Verification items for this drawing (mm, ordinates from the low corner). A direction names the side the tool comes from. Round coordinates to 2 decimals unless told otherwise and drop trailing zeros. Loops run counter-clockwise (first coordinate to the right, second up) from the corner with the lowest first, then second, coordinate; pieces in that order, holes last. Notation, with made-up numbers: (83.25, 12.5) -> (108.25, 12.5) arc R8 cw to (108.25, 21.5) -> close; hole circle Ø3 at (-7.75, 82). An arc over 180 degrees is marked (long way). One line per item, written item: value. Start each with the question number.
1. Cross-section at D-D on z = 41.5. Record the cut outline in (x, y), then the cut area to 3 significant figures.
2. Cross-section at C-C on z = 66. Record the cut outline in (x, y).
3. Material ranges on L1, parallel to Z at x = 33.5, y = 19.5; L2, parallel to X at y = 18, z = 29 (3 decimals); L3, parallel to Y at x = 28, z = 39, recorded low to high.
4. Go/stop test with flat-tipped pins: pin 1 (3 mm diameter, centred on x = 30, z = 19.5, fed in from +Y); pin 2 (5 mm diameter, centred on x = 11.5, y = 20.5, fed in from -Z); pin 3 (6 mm diameter, centred on x = 20.5, z = 18, fed in from +Y); pin 4 (4 mm diameter, centred on y = 25.5, z = 58, fed in from -X). Record where each tip stops, or that it passes through.
5. Set-up check for the marked faces 1, 2 and 3: record each of +Z, -Z, +X, -X, +Y, -Y from which the full face is reachable in a straight line by a thin tool's end or side.
6. Cross-section at A-A on x = 18.75. Record the cut outline in (y, z), then the cut area to 3 significant figures.
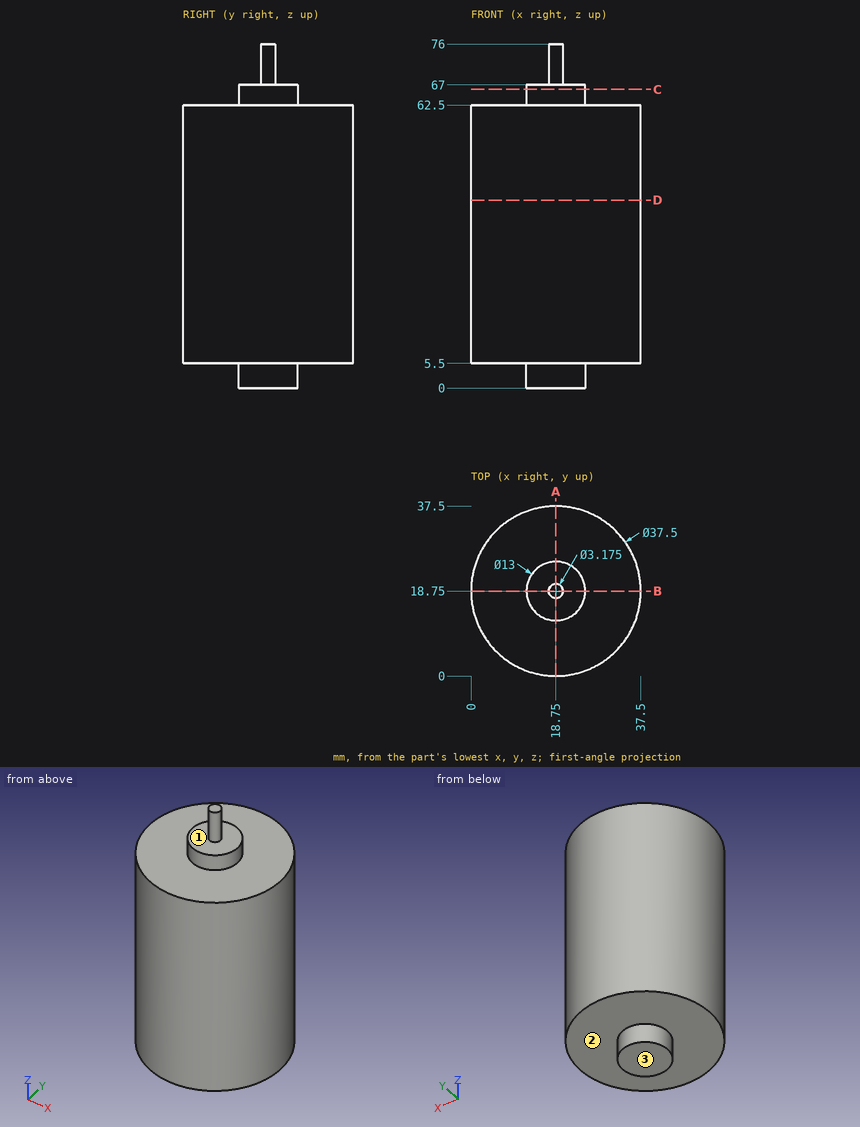
Taken from the geometry:
1. outline: circle Ø37.5 at (18.75, 18.75)
1. area: 1,100 mm2
2. outline: circle Ø13 at (18.75, 18.75)
3. L1: z = 5.5 to 62.5
3. L2: x = 0.015 to 37.485
3. L3: y = 2.44 to 35.06
4. pin 1: stops at y = 34.77
4. pin 2: stops at z = 0
4. pin 3: stops at y = 37.5
4. pin 4: stops at x = 0.61
5. face 1: +Z
5. face 2: -Z
5. face 3: -Z, +X, -X, +Y, -Y
6. outline: (0, 5.5) -> (12.25, 5.5) -> (12.25, 0) -> (25.25, 0) -> (25.25, 5.5) -> (37.5, 5.5) -> (37.5, 62.5) -> (25.25, 62.5) -> (25.25, 67) -> (20.34, 67) -> (20.34, 76) -> (17.16, 76) -> (17.16, 67) -> (12.25, 67) -> (12.25, 62.5) -> (0, 62.5) -> close
6. area: 2,300 mm2
